Work out the finished part from the listing and answer in its coordinate system (mm). A direction names the side the tool comes from. Give positions to 0.01 mm unless a question says otherwise; leave off trailing zeros. Order: outer loops, then holes, each group sorted by start corner. A loop starts at its lowest first (then second) coordinate and runs counter-clockwise, first axis right, second up. Notation, with made-up numbers: (-17, 4.5) - (4, 4.5) arc R19 ccw to (4, 9.5) - close; hole circle Ø9 at (67.5, 21.5). An arc over 180 degrees is marked (long way). Write each question's results on one line, items separated by ' | '.
from build123d import *

# Parameters (mm, degrees)
SKETCH6_W               = 4
SKETCH6_H               = 4
SKETCH8_R               = 1.5
BOSS_EXTRUDE4_DEPTH     = 3
SKETCH9_W               = 4
SKETCH9_H               = 4
BOSS_EXTRUDE5_DEPTH     = 10
CUT_EXTRUDE1_DEPTH      = 11.954451205
CUT_EXTRUDE1_DEPTH_BACK = 11.954451205
CUT_EXTRUDE_THIN1_DEPTH = 10
SKETCH12_R              = 0.625
CUT_EXTRUDE2_DEPTH      = 11.954451205
CUT_EXTRUDE2_DEPTH_BACK = 11.954451205
SKETCH13_R              = 1
CUT_EXTRUDE3_DEPTH      = 18.233687963
CUT_EXTRUDE3_DEPTH_BACK = 18.233687963
SKETCH14_R              = 1.920216589
BOSS_EXTRUDE6_DEPTH     = 0.5
SKETCH15_R              = 0.625
BOSS_EXTRUDE7_DEPTH     = 3


with BuildPart() as part:
    # Sketch7 for Loft1 → Loft1 section 0
    with BuildSketch(Plane(origin=(0, 4, 0), x_dir=(1, 0, 0), z_dir=(0, 1, 0))):
        with BuildLine():
            # circular arc as an exact rational Bezier (weights 1, cos(half-angle), 1)
            Bezier((-1.060660172, -1.060660172), (0, -2.121320343), (1.060660172, -1.060660172), weights=[1, 0.707106782, 1])
            Bezier((1.060660172, -1.060660172), (2.121320343, 0), (1.060660172, 1.060660172), weights=[1, 0.707106782, 1])
            Bezier((1.060660172, 1.060660172), (0, 2.121320343), (-1.060660172, 1.060660172), weights=[1, 0.707106782, 1])
            Bezier((-1.060660172, 1.060660172), (-2.121320343, 0), (-1.060660172, -1.060660172), weights=[1, 0.707106782, 1])
        make_face()
    # Sketch6 → Loft1 section 1
    with BuildSketch(Plane(origin=(0, 0, 0), x_dir=(1, 0, 0), z_dir=(0, 1, 0))):
        Rectangle(SKETCH6_W, SKETCH6_H)
    loft()

    # Sketch8 → Boss-Extrude4 (add)
    with BuildSketch(Plane(origin=(0, 4, 0), x_dir=(1, 0, 0), z_dir=(0, 1, 0))):
        with Locations(Location((0, 0, 0), (0, 0, 45))):
            Circle(SKETCH8_R)
    extrude(amount=BOSS_EXTRUDE4_DEPTH)

    # Sketch9 → Boss-Extrude5 (add)
    with BuildSketch(Plane.XZ):
        Rectangle(SKETCH9_W, SKETCH9_H)
    extrude(amount=BOSS_EXTRUDE5_DEPTH)

    # Sketch10 → Cut-Extrude1 (cut, two sides)
    with BuildSketch(Plane(origin=(0, 0, -2), x_dir=(-1, 0, 0), z_dir=(0, 0, -1))) as cut_extrude1_sk:
        with BuildLine():
            Line((-1.5, -10), (-1.5, 0))
            add(Edge.make_bspline(
                [(-1.5, 0), (0, 7), (1.5, 0)],
                knots=[0, 0, 0, 1, 1, 1], degree=2, weights=[1, 1.333333333, 1]))
            Line((1.5, 0), (1.5, -10))
            Line((1.5, -10), (-1.5, -10))
        make_face()
    extrude(amount=CUT_EXTRUDE1_DEPTH, mode=Mode.SUBTRACT)
    extrude(cut_extrude1_sk.sketch, amount=-CUT_EXTRUDE1_DEPTH_BACK, mode=Mode.SUBTRACT)

    # Sketch11 → Cut-Extrude-Thin1 (cut)
    with BuildSketch(Plane(origin=(2, 0, 0), x_dir=(0, 0, -1), z_dir=(1, 0, 0))):
        with BuildLine():
            Line((11.997667212, -7.763395965), (11.17222068, 17))
            Line((11.17222068, 17), (-11.17222068, 17))
            Line((-11.17222068, 17), (-11.997667212, -7.763395965))
            ThreePointArc((-11.997667212, -7.763395965), (0, -20), (11.997667212, -7.763395965))
        make_face()
        with BuildLine():
            Line((2, -8), (1.5, 7))
            Line((1.5, 7), (-1.5, 7))
            Line((-1.5, 7), (-2, -8))
            ThreePointArc((-2, -8), (0, -10), (2, -8))
        make_face(mode=Mode.SUBTRACT)
    extrude(amount=-CUT_EXTRUDE_THIN1_DEPTH, mode=Mode.SUBTRACT)

    # Sketch12 → Cut-Extrude2 (cut, two sides)
    with BuildSketch(Plane(origin=(2, 0, 0), x_dir=(0, 0, -1), z_dir=(1, 0, 0))) as cut_extrude2_sk:
        with Locations((0, -8.079783411)):
            Circle(SKETCH12_R)
    extrude(amount=CUT_EXTRUDE2_DEPTH, mode=Mode.SUBTRACT)
    extrude(cut_extrude2_sk.sketch, amount=-CUT_EXTRUDE2_DEPTH_BACK, mode=Mode.SUBTRACT)

    # Sketch13 → Cut-Extrude3 (cut, two sides)
    with BuildSketch(Plane(origin=(0, 7, 0), x_dir=(1, 0, 0), z_dir=(0, 1, 0))) as cut_extrude3_sk:
        with Locations(Location((0, 0, 0), (0, 0, 270))):
            Circle(SKETCH13_R)
    extrude(amount=CUT_EXTRUDE3_DEPTH, mode=Mode.SUBTRACT)
    extrude(cut_extrude3_sk.sketch, amount=-CUT_EXTRUDE3_DEPTH_BACK, mode=Mode.SUBTRACT)

    # Sketch14 → Boss-Extrude6 (add)
    with BuildSketch(Plane(origin=(-1.5, 0, 0), x_dir=(0, 0, -1), z_dir=(1, 0, 0))):
        with Locations(Location((0, -8.079783411, 0), (0, 0, 269.997072333))):
            Circle(SKETCH14_R)
    extrude(amount=BOSS_EXTRUDE6_DEPTH)

    # Sketch15 → Boss-Extrude7 (add)
    with BuildSketch(Plane(origin=(-1, 0, 0), x_dir=(0, 0, -1), z_dir=(1, 0, 0))):
        with Locations((0, -8.079783411)):
            Circle(SKETCH15_R)
    extrude(amount=BOSS_EXTRUDE7_DEPTH)


solid = part.part
1. Determine the mould class of faces 1 (the face through (0.806, 5.479, 1.265)), 2 (the face through (-1.75, -8.69, 0.14)), 3 (the face through (1.5, -5, 0)), 4 (the face through (-1.7, -10, 0)) for opening direction Y: +Y half, -Y half, draft (parallel to the pull), parting line (faces both ways), or undercut.
Answer list:
face 1: draft | face 2: undercut | face 3: undercut | face 4: -Y half
2. A tool of negligible diameter and unlimited length cuts with its end or side. For faces 5 (the face through (0, 5, -1)), 6 (the face through (-1, -8, 1)), 7 (the face through (2, -5, 0)), 8 (the face through (-1.5, -8, 0)), from which of +Z, -Z, +X, -X, +Y, -Y can it reach the whole face along a straight path? Write none if from no direction.
Answer list:
face 5: +Y | face 6: none | face 7: +Z, -Z, +X, +Y, -Y | face 8: -X
3. Given P1, Ø1, axis at y = 4.5, z = -1, coming from the -X side; P2, Ø1, axis at y = -8, z = 0, coming from the -X side; P3, Ø1.8, axis at x = 0, z = 0, coming from the +Y side, each flat-ended and moving along its own axis, determine where each tip first touches the part or whether it passes through.
Answer list:
P1: x = -1.41 | P2: x = -1.5 | P3: y = -7.45
4. A cutting plane is placed at B-B, the plane y = -8.5. Write down the section's boundary in (x, z).
Answer list:
outline: (-2, -1.94) - (-1.5, -1.94) - (-1.5, -1.87) - (-1, -1.87) - (-1, -0.46) - (1.5, -0.46) - (1.5, -1.94) - (2, -1.94) - (2, 1.94) - (1.5, 1.94) - (1.5, 0.46) - (-1, 0.46) - (-1, 1.87) - (-1.5, 1.87) - (-1.5, 1.94) - (-2, 1.94) - (-2, 0.46) - (-1.5, 0.46) - (-1.5, -0.46) - (-2, -0.46) - close
5. A cutting plane is placed at A-A, the plane y = 4.25. Write down the section's boundary in (x, z), then the cut area to 3 significant figures.
Answer list:
outline: circle Ø3 at (0, 0); hole circle Ø2 at (0, 0) | area: 3.93 mm^2
6. A cutting plane is placed at C-C, the plane x = 0.5. State how many separate pieces and enclosed holes the cut face has, then the cut area to 3 significant figures.
Answer list:
separate pieces: 3 | enclosed holes: 0 | area: 5.12 mm^2
7. Straight lines are drawn through the part: line 1 (X direction, y = -5.5, z = 1.5); line 2 (X direction, y = 4, z = 0); line 3 (Z direction, x = 0.8, y = 4). For each, find the intervals that lie inside material, in ascending order. Write a range as [from, to].
Answer list:
line 1: [-2, -1.5], [1.5, 2] | line 2: [-1.5, -1], [1, 1.5] | line 3: [-1.27, -0.6], [0.6, 1.27]
